Geometry check sheet. Reference: drawing and pictorial views, mm from the part's lowest x, y, z. A direction names the side the tool comes from. Give positions to 0.01 mm unless a question says otherwise; leave off trailing zeros. Write each loop counter-clockwise with the first axis right and the second up, starting at its lowest first coordinate (ties: lowest second). Pieces come first, ordered by that corner, then holes. Notation, with made-up numbers: (-6, 21.5) -> (6, 21.5) arc R37 cw to (6, 58.5) -> close; hole circle Ø11 at (7, -8). An arc over 180 degrees is marked (long way). Use a Markdown table: item, result. Add a question column.
1. Cross-section at A-A (x = 5.65). Enter the section's corners in (y, z) (3 decimals).
2. Cross-section at D-D (y = 20). Enter the section's corners in (x, z), then the cut area to 3 significant figures.
3. Release check for a two-part mould opening along Z. For the marked faces 1, 2 and 3 record: released by +Z, released by -Z, zero draft, split by the parting line, or undercut.
4. Gauge pin test, flat ends, axial feed: P1, Ø2.5, axis at x = 3, z = 1.5, coming from the +Y side; P2, Ø1.5, axis at x = 37, z = 1, coming from the +Y side; P3, Ø2.5, axis at x = 36.65, y = 8.65, coming from the -Z side. Record the tip position at first contact, or that the pin passes through.
5. Cross-section at B-B (y = 36.5). Enter the section's corners in (x, z), then the cut area to 3 significant figures.
6. Cross-section at C-C (z = 39.5). Enter the section's corners in (x, y), then the cut area to 3 significant figures.
7. Scan lines: probe 1 along Z at (x, y) = (24.5, 12.5); probe 2 along Y at (x, z) = (17, 38); probe 3 along Y at (x, z) = (5.65, 1.1) (3 decimals). Record each from-to range of solid material in increasing order. Write a range as [from, to].
8. Set-up check for the marked faces 4 and 5: record each of +Z, -Z, +X, -X, +Y, -Y from which the full face is reachable in a straight line by a thin tool's end or side.
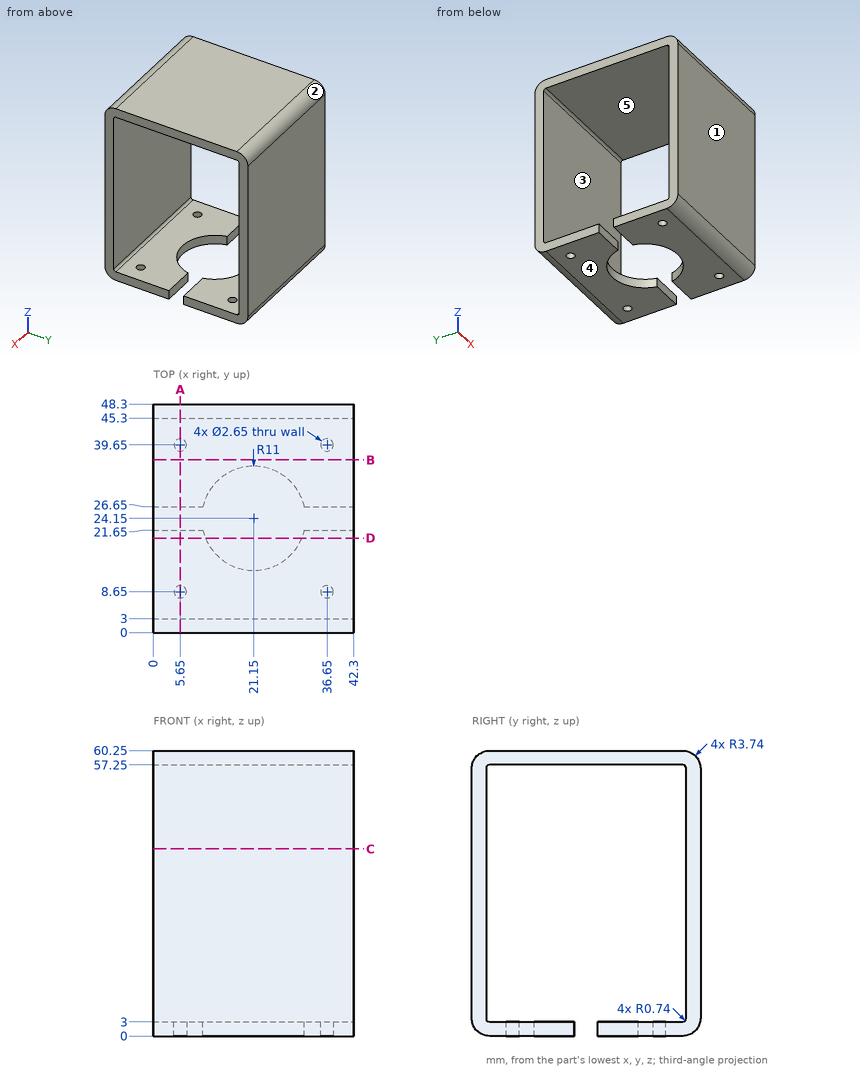
Worked answers:
| question | item | result |
|---|---|---|
| 1 | outline | (0, 3.74) arc R3.74 ccw to (3.74, 0) -> (7.325, 0) -> (7.325, 3) -> (3.74, 3) arc R0.74 cw to (3, 3.74) -> (3, 56.51) arc R0.74 cw to (3.74, 57.25) -> (44.56, 57.25) arc R0.74 cw to (45.3, 56.51) -> (45.3, 3.74) arc R0.74 cw to (44.56, 3) -> (40.975, 3) -> (40.975, 0) -> (44.56, 0) arc R3.74 ccw to (48.3, 3.74) -> (48.3, 56.51) arc R3.74 ccw to (44.56, 60.25) -> (3.74, 60.25) arc R3.74 ccw to (0, 56.51) -> close; (9.975, 0) -> (21.65, 0) -> (21.65, 3) -> (9.975, 3) -> close; (26.65, 0) -> (38.325, 0) -> (38.325, 3) -> (26.65, 3) -> close |
| 2 | outline | (0, 0) -> (10.96, 0) -> (10.96, 3) -> (0, 3) -> close; (0, 57.25) -> (42.3, 57.25) -> (42.3, 60.25) -> (0, 60.25) -> close; (31.34, 0) -> (42.3, 0) -> (42.3, 3) -> (31.34, 3) -> close |
| 2 | area | 193 mm² |
| 3 | face 1 | zero draft |
| 3 | face 2 | released by +Z |
| 3 | face 3 | undercut |
| 4 | P1 | stops at y = 48.17 |
| 4 | P2 | stops at y = 47.73 |
| 4 | P3 | stops at z = 57.25 |
| 5 | outline | (0, 0) -> (42.3, 0) -> (42.3, 3) -> (0, 3) -> close; (0, 57.25) -> (42.3, 57.25) -> (42.3, 60.25) -> (0, 60.25) -> close |
| 5 | area | 254 mm² |
| 6 | outline | (0, 0) -> (42.3, 0) -> (42.3, 3) -> (0, 3) -> close; (0, 45.3) -> (42.3, 45.3) -> (42.3, 48.3) -> (0, 48.3) -> close |
| 6 | area | 254 mm² |
| 7 | probe 1 | z = [0, 3], [57.25, 60.25] |
| 7 | probe 2 | y = [0, 3], [45.3, 48.3] |
| 7 | probe 3 | y = [1.091, 7.325], [9.975, 21.65], [26.65, 38.325], [40.975, 47.209] |
| 8 | face 4 | -Z, +X, -X, +Y, -Y |
| 8 | face 5 | +X, -X |
